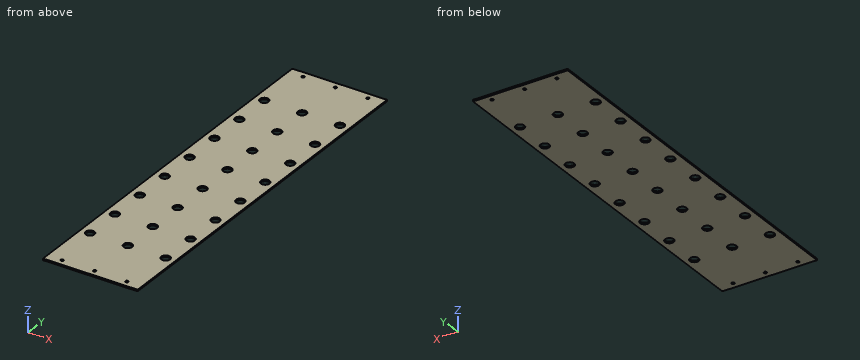
from build123d import *

# Parameters (mm, degrees)
SKETCH1_W        = 280.02
SKETCH1_H        = 1122
PLATE_DEPTH      = 4.76
HOLES_DEPTH      = 1157.424601087
HOLES_DEPTH_BACK = 1157.424601087
SKETCH2_R        = 4.37
SKETCH2_R_2      = 13


with BuildPart() as part:
    # Sketch1 → Plate (new body)
    with BuildSketch(Plane.XY):
        with Locations((140.01, 561)):
            Rectangle(SKETCH1_W, SKETCH1_H)
    extrude(amount=PLATE_DEPTH)

    # Sketch2 → Holes (cut, two sides: drawn at the far end of the back side and taken through both)
    with BuildSketch(Plane.XY.offset(-HOLES_DEPTH_BACK)):
        with Locations((44.06, 19.05)):
            Circle(SKETCH2_R)
        with Locations((44.06, 1102.95)):
            Circle(SKETCH2_R)
        with Locations((140.01, 19.05)):
            Circle(SKETCH2_R)
        with Locations((140.01, 1102.95)):
            Circle(SKETCH2_R)
        with Locations((235.96, 19.05)):
            Circle(SKETCH2_R)
        with Locations((235.96, 1102.95)):
            Circle(SKETCH2_R)
        with Locations((28.01, 169)):
            Circle(SKETCH2_R_2)
        with Locations((28.01, 281)):
            Circle(SKETCH2_R_2)
        with Locations((28.01, 393)):
            Circle(SKETCH2_R_2)
        with Locations((28.01, 505)):
            Circle(SKETCH2_R_2)
        with Locations((28.01, 617)):
            Circle(SKETCH2_R_2)
        with Locations((28.01, 729)):
            Circle(SKETCH2_R_2)
        with Locations((28.01, 841)):
            Circle(SKETCH2_R_2)
        with Locations((28.01, 953)):
            Circle(SKETCH2_R_2)
        with Locations((140.01, 169)):
            Circle(SKETCH2_R_2)
        with Locations((140.01, 281)):
            Circle(SKETCH2_R_2)
        with Locations((140.01, 393)):
            Circle(SKETCH2_R_2)
        with Locations((140.01, 505)):
            Circle(SKETCH2_R_2)
        with Locations((140.01, 617)):
            Circle(SKETCH2_R_2)
        with Locations((140.01, 729)):
            Circle(SKETCH2_R_2)
        with Locations((140.01, 841)):
            Circle(SKETCH2_R_2)
        with Locations((140.01, 953)):
            Circle(SKETCH2_R_2)
        with Locations((252.01, 169)):
            Circle(SKETCH2_R_2)
        with Locations((252.01, 281)):
            Circle(SKETCH2_R_2)
        with Locations((252.01, 393)):
            Circle(SKETCH2_R_2)
        with Locations((252.01, 505)):
            Circle(SKETCH2_R_2)
        with Locations((252.01, 617)):
            Circle(SKETCH2_R_2)
        with Locations((252.01, 729)):
            Circle(SKETCH2_R_2)
        with Locations((252.01, 841)):
            Circle(SKETCH2_R_2)
        with Locations((252.01, 953)):
            Circle(SKETCH2_R_2)
    extrude(amount=HOLES_DEPTH + HOLES_DEPTH_BACK, mode=Mode.SUBTRACT)


solid = part.part
Part model, mm, in its own coordinate system. Give positions to 0.01 mm unless a question says otherwise; leave off trailing zeros. Loops run counter-clockwise (first coordinate to the right, second up) from the corner with the lowest first, then second, coordinate; pieces in that order, holes last. Notation, with made-up numbers: M 61,16 L 100,16 A30 ccw 100,55 Z; hole C 5,8.25 d10. An arc over 180 degrees is marked long. Put each result on its own line as item: value. Start each with the question number.
1) Saw through at A-A (z = 3). State how many separate pieces and enclosed holes the cut face has, then the cut area to 3 significant figures.
2) Saw through at B-B (y = 505). List the corners of the cut face in (x, z).
3) Probe probe 1 along X at (y, z) = (953, 2.6); probe 2 along Y at (x, z) = (235.96, 1.4); probe 3 along X at (y, z) = (495, 4). List the from-to ranges inside material, lowest first.
4) Flat gauge pins, fed straight in: pin 1 (21 mm diameter, centred on x = 252.01, y = 841, fed in from -Z); pin 2 (4 mm diameter, centred on x = 150, y = 253, fed in from -Z). Where does each tip first touch, or does it go through?
Numbers:
1. separate pieces: 1
1. enclosed holes: 30
1. area: 301,000 mm^2
2. outline: M 0,0 L 15.01,0 L 15.01,4.76 L 0,4.76 Z; M 41.01,0 L 127.01,0 L 127.01,4.76 L 41.01,4.76 Z; M 153.01,0 L 239.01,0 L 239.01,4.76 L 153.01,4.76 Z; M 265.01,0 L 280.02,0 L 280.02,4.76 L 265.01,4.76 Z
3. probe 1: 0 to 15.01, 41.01 to 127.01, 153.01 to 239.01, 265.01 to 280.02
3. probe 2: 0 to 14.68, 23.42 to 1098.58, 1107.32 to 1122
3. probe 3: 0 to 19.7, 36.32 to 131.7, 148.32 to 243.7, 260.32 to 280.02
4. pin 1: through
4. pin 2: z = 0
